Verification items for the finished model (mm, model axes). A direction names the side the tool comes from. Coordinates: 2 decimals unless noted, no trailing zeros. Write each loop counter-clockwise with the first axis right and the second up, starting at its lowest first coordinate (ties: lowest second). Pieces come first, ordered by that corner, then holes. Notation, with made-up numbers: (69.25, -26) -> (128.25, -26) arc R34 ccw to (128.25, 13) -> close; hole circle Ø8 at (20.25, -7). An arc over 180 degrees is marked (long way). Answer in a Markdown table with one row per item.
```python
from build123d import *

# Parameters (mm, degrees)
EXTRUDE_F_DEPTH    = 736.6
CUT_EXTRUDE1_REACH = 5.175
SKETCH2_R          = 2.667
CUT_EXTRUDE2_REACH = 5.175
SKETCH3_R          = 2.667


with BuildPart() as part:
    # Sketch1 → Extrude f (new body)
    with BuildSketch(Plane.XY):
        Polygon((3.175, 3.175), (3.175, 25.4), (0, 25.4), (0, 0), (50.8, 0), (50.8, 25.4), (47.625, 25.4), (47.625, 3.175), align=None)
    extrude(amount=EXTRUDE_F_DEPTH)

    # Sketch2 → Cut-Extrude1 (cut, up to next)
    with BuildSketch(Plane(origin=(0, 3.175, 0), x_dir=(1, 0, 0), z_dir=(0, 1, 0)), mode=Mode.PRIVATE) as cut_extrude1_sk1:
        with Locations((12.7, -723.9)):
            Circle(SKETCH2_R)
    cut_extrude1_tool1 = extrude(cut_extrude1_sk1.sketch, amount=-CUT_EXTRUDE1_REACH, mode=Mode.PRIVATE) & part.part
    add(cut_extrude1_tool1.solids().sort_by_distance((12.7, 3.175, 723.9))[0], mode=Mode.SUBTRACT)
    # Sketch2 → Cut-Extrude1 (cut, up to next)
    with BuildSketch(Plane(origin=(0, 3.175, 0), x_dir=(1, 0, 0), z_dir=(0, 1, 0)), mode=Mode.PRIVATE) as cut_extrude1_sk2:
        with Locations((12.7, -660.4)):
            Circle(SKETCH2_R)
    cut_extrude1_tool2 = extrude(cut_extrude1_sk2.sketch, amount=-CUT_EXTRUDE1_REACH, mode=Mode.PRIVATE) & part.part
    add(cut_extrude1_tool2.solids().sort_by_distance((12.7, 3.175, 660.4))[0], mode=Mode.SUBTRACT)
    # Sketch2 → Cut-Extrude1 (cut, up to next)
    with BuildSketch(Plane(origin=(0, 3.175, 0), x_dir=(1, 0, 0), z_dir=(0, 1, 0)), mode=Mode.PRIVATE) as cut_extrude1_sk3:
        with Locations((38.1, -660.4)):
            Circle(SKETCH2_R)
    cut_extrude1_tool3 = extrude(cut_extrude1_sk3.sketch, amount=-CUT_EXTRUDE1_REACH, mode=Mode.PRIVATE) & part.part
    add(cut_extrude1_tool3.solids().sort_by_distance((38.1, 3.175, 660.4))[0], mode=Mode.SUBTRACT)
    # Sketch2 → Cut-Extrude1 (cut, up to next)
    with BuildSketch(Plane(origin=(0, 3.175, 0), x_dir=(1, 0, 0), z_dir=(0, 1, 0)), mode=Mode.PRIVATE) as cut_extrude1_sk4:
        with Locations((38.1, -723.9)):
            Circle(SKETCH2_R)
    cut_extrude1_tool4 = extrude(cut_extrude1_sk4.sketch, amount=-CUT_EXTRUDE1_REACH, mode=Mode.PRIVATE) & part.part
    add(cut_extrude1_tool4.solids().sort_by_distance((38.1, 3.175, 723.9))[0], mode=Mode.SUBTRACT)
    # Sketch2 → Cut-Extrude1 (cut, up to next)
    with BuildSketch(Plane(origin=(0, 3.175, 0), x_dir=(1, 0, 0), z_dir=(0, 1, 0)), mode=Mode.PRIVATE) as cut_extrude1_sk5:
        with Locations((38.1, -12.7)):
            Circle(SKETCH2_R)
    cut_extrude1_tool5 = extrude(cut_extrude1_sk5.sketch, amount=-CUT_EXTRUDE1_REACH, mode=Mode.PRIVATE) & part.part
    add(cut_extrude1_tool5.solids().sort_by_distance((38.1, 3.175, 12.7))[0], mode=Mode.SUBTRACT)
    # Sketch2 → Cut-Extrude1 (cut, up to next)
    with BuildSketch(Plane(origin=(0, 3.175, 0), x_dir=(1, 0, 0), z_dir=(0, 1, 0)), mode=Mode.PRIVATE) as cut_extrude1_sk6:
        with Locations((38.1, -76.2)):
            Circle(SKETCH2_R)
    cut_extrude1_tool6 = extrude(cut_extrude1_sk6.sketch, amount=-CUT_EXTRUDE1_REACH, mode=Mode.PRIVATE) & part.part
    add(cut_extrude1_tool6.solids().sort_by_distance((38.1, 3.175, 76.2))[0], mode=Mode.SUBTRACT)
    # Sketch2 → Cut-Extrude1 (cut, up to next)
    with BuildSketch(Plane(origin=(0, 3.175, 0), x_dir=(1, 0, 0), z_dir=(0, 1, 0)), mode=Mode.PRIVATE) as cut_extrude1_sk7:
        with Locations((12.7, -12.7)):
            Circle(SKETCH2_R)
    cut_extrude1_tool7 = extrude(cut_extrude1_sk7.sketch, amount=-CUT_EXTRUDE1_REACH, mode=Mode.PRIVATE) & part.part
    add(cut_extrude1_tool7.solids().sort_by_distance((12.7, 3.175, 12.7))[0], mode=Mode.SUBTRACT)
    # Sketch2 → Cut-Extrude1 (cut, up to next)
    with BuildSketch(Plane(origin=(0, 3.175, 0), x_dir=(1, 0, 0), z_dir=(0, 1, 0)), mode=Mode.PRIVATE) as cut_extrude1_sk8:
        with Locations((12.7, -76.2)):
            Circle(SKETCH2_R)
    cut_extrude1_tool8 = extrude(cut_extrude1_sk8.sketch, amount=-CUT_EXTRUDE1_REACH, mode=Mode.PRIVATE) & part.part
    add(cut_extrude1_tool8.solids().sort_by_distance((12.7, 3.175, 76.2))[0], mode=Mode.SUBTRACT)

    # Sketch3 → Cut-Extrude2 (cut, up to next)
    with BuildSketch(Plane(origin=(0, 3.175, 0), x_dir=(1, 0, 0), z_dir=(0, 1, 0)), mode=Mode.PRIVATE) as cut_extrude2_sk1:
        with Locations((34.925, -207.9371)):
            Circle(SKETCH3_R)
    cut_extrude2_tool1 = extrude(cut_extrude2_sk1.sketch, amount=-CUT_EXTRUDE2_REACH, mode=Mode.PRIVATE) & part.part
    add(cut_extrude2_tool1.solids().sort_by_distance((34.925, 3.175, 207.9371))[0], mode=Mode.SUBTRACT)
    # Sketch3 → Cut-Extrude2 (cut, up to next)
    with BuildSketch(Plane(origin=(0, 3.175, 0), x_dir=(1, 0, 0), z_dir=(0, 1, 0)), mode=Mode.PRIVATE) as cut_extrude2_sk2:
        with Locations((15.875, -207.9371)):
            Circle(SKETCH3_R)
    cut_extrude2_tool2 = extrude(cut_extrude2_sk2.sketch, amount=-CUT_EXTRUDE2_REACH, mode=Mode.PRIVATE) & part.part
    add(cut_extrude2_tool2.solids().sort_by_distance((15.875, 3.175, 207.9371))[0], mode=Mode.SUBTRACT)
    # Sketch3 → Cut-Extrude2 (cut, up to next)
    with BuildSketch(Plane(origin=(0, 3.175, 0), x_dir=(1, 0, 0), z_dir=(0, 1, 0)), mode=Mode.PRIVATE) as cut_extrude2_sk3:
        with Locations((34.925, -182.5371)):
            Circle(SKETCH3_R)
    cut_extrude2_tool3 = extrude(cut_extrude2_sk3.sketch, amount=-CUT_EXTRUDE2_REACH, mode=Mode.PRIVATE) & part.part
    add(cut_extrude2_tool3.solids().sort_by_distance((34.925, 3.175, 182.5371))[0], mode=Mode.SUBTRACT)
    # Sketch3 → Cut-Extrude2 (cut, up to next)
    with BuildSketch(Plane(origin=(0, 3.175, 0), x_dir=(1, 0, 0), z_dir=(0, 1, 0)), mode=Mode.PRIVATE) as cut_extrude2_sk4:
        with Locations((15.875, -182.5371)):
            Circle(SKETCH3_R)
    cut_extrude2_tool4 = extrude(cut_extrude2_sk4.sketch, amount=-CUT_EXTRUDE2_REACH, mode=Mode.PRIVATE) & part.part
    add(cut_extrude2_tool4.solids().sort_by_distance((15.875, 3.175, 182.5371))[0], mode=Mode.SUBTRACT)


solid = part.part
```
1. Sectioned sample at B-B, the plane z = 555.5. Record the cut outline in (x, y) (3 decimals).
Findings below:
| item | result |
|---|---|
| outline | (0, 0) -> (50.8, 0) -> (50.8, 25.4) -> (47.625, 25.4) -> (47.625, 3.175) -> (3.175, 3.175) -> (3.175, 25.4) -> (0, 25.4) -> close |
2. Material ranges on probe 1 along Z at (x, y) = (38.1, 1.1); probe 2 along X at (y, z) = (1.25, 76.2); probe 3 along X at (y, z) = (19, 299) (3 decimals), recorded low to high. Write a range as from..to.
Findings below:
| item | result |
|---|---|
| probe 1 | z = 0..10.03, 15.37..73.53, 78.87..657.73, 663.07..721.23, 726.57..736.6 |
| probe 2 | x = 0..10.03, 15.37..35.43, 40.77..50.8 |
| probe 3 | x = 0..3.175, 47.625..50.8 |
3. Sectioned sample at A-A, the plane y = 13.5. Record the cut outline in (x, z) (3 decimals), and give its area (3 significant figures).
Findings below:
| item | result |
|---|---|
| outline | (0, 0) -> (3.175, 0) -> (3.175, 736.6) -> (0, 736.6) -> close; (47.625, 0) -> (50.8, 0) -> (50.8, 736.6) -> (47.625, 736.6) -> close |
| area | 4,680 mm² |
4. Go/stop test with flat-tipped pins: pin 1 (4 mm diameter, centred on x = 15.5, z = 149, fed in from +Y) (3 decimals); pin 2 (3 mm diameter, centred on x = 13, z = 606.5, fed in from -Y). Record where each tip stops, or that it passes through.
Findings below:
| item | result |
|---|---|
| pin 1 | stops at y = 3.175 |
| pin 2 | stops at y = 0 |
5. Access from +Z, -Z, +X, -X, +Y, -Y to the whole of each face (thin tool, end or side, straight path). Record for faces 1 (the face through (50.8, 13, 363)), 2 (the face through (26, 3.175, 363)).
Findings below:
| item | result |
|---|---|
| face 1 | +Z, -Z, +X, +Y, -Y |
| face 2 | +Z, -Z, +Y |
6. Release check for a two-part mould opening along X. For faces 3 (the face through (0, 13, 363)), 4 (the face through (47.625, 14, 363)), 5 (the face through (27, 2, 0)) record: released by +X, released by -X, zero draft, split by the parting line, or undercut.
Findings below:
| item | result |
|---|---|
| face 3 | released by -X |
| face 4 | undercut |
| face 5 | zero draft |
